CAD build for the part. Positions are in the model's coordinates, mm. A direction names the side the tool comes from. Coordinates: 2 decimals unless noted, no trailing zeros. Order: outer loops, then holes, each group sorted by start corner. A loop starts at its lowest first (then second) coordinate and runs counter-clockwise, first axis right, second up. Notation, with made-up numbers: M 23,57.25 L 40,57.25 A22 cw 40,76.25 Z; hole C 45.5,-1.75 d4. An arc over 180 degrees is marked long. One line per item, written item: value.
from build123d import *

# Parameters (mm, degrees)
SKETCH2_R                = 3.175
CUT_EXTRUDE1_DEPTH       = 6.715
CUT_EXTRUDE1_DEPTH_BACK  = 6.715
SKETCH3_R                = 5.715
SKETCH3_R_2              = 3.175
BOSS_EXTRUDE1_DEPTH      = 6.0325
BOSS_EXTRUDE1_DEPTH_BACK = 6.0325
SKETCH4_W                = 5.08
SKETCH4_H                = 5.08
BOSS_EXTRUDE2_DEPTH      = 25.4


with BuildPart() as part:
    # Sketch1 → Revolve1 (revolve)
    with BuildSketch(Plane.XY):
        with BuildLine():
            Line((0, 5.715), (0, -5.715))
            ThreePointArc((0, -5.715), (5.715, 0), (0, 5.715))
        make_face()
    revolve(axis=Axis((0, 5.715, 0), (0, -1, 0)))

    # Sketch2 → Cut-Extrude1 (cut, two sides)
    with BuildSketch(Plane(origin=(0, 0, 0), x_dir=(1, 0, 0), z_dir=(0, 1, 0))) as cut_extrude1_sk:
        Circle(SKETCH2_R)
    extrude(amount=CUT_EXTRUDE1_DEPTH, mode=Mode.SUBTRACT)
    extrude(cut_extrude1_sk.sketch, amount=-CUT_EXTRUDE1_DEPTH_BACK, mode=Mode.SUBTRACT)

    # Sketch3 → Boss-Extrude1 (add, two sides)
    with BuildSketch(Plane(origin=(0, 0, 0), x_dir=(1, 0, 0), z_dir=(0, 1, 0))) as boss_extrude1_sk:
        Circle(SKETCH3_R)
        Circle(SKETCH3_R_2, mode=Mode.SUBTRACT)
    extrude(amount=BOSS_EXTRUDE1_DEPTH)
    extrude(boss_extrude1_sk.sketch, amount=-BOSS_EXTRUDE1_DEPTH_BACK)

    # Sketch4 → Boss-Extrude2 (add)
    with BuildSketch(Plane(origin=(0, 0, 0), x_dir=(0, 0, -1), z_dir=(-0.993884104, 0.1104282, 0))):
        Rectangle(SKETCH4_W, SKETCH4_H)
    extrude(amount=-BOSS_EXTRUDE2_DEPTH)


solid = part.part
Q1. Slice it at D-D (y = 5.5). List the corners of the cut face in (x, z) (3 decimals).
Recorded:
outline: C 0,0 d11.43; hole C 0,0 d6.35
Q2. Which spindle directions (+Z, -Z, +X, -X, +Y, -Y) get a long thin tool onto all of the face, cutting with end or side? Do faces 1 (the face through (0, 0, 0)), 2 (the face through (1.423, -2.714, 0.036)), 3 (the face through (15, -2, 2.54)), 4 (the face through (15, -2, -2.54)), 5 (the face through (2.5, 6.032, 2.5)). Say none if no direction does.
Recorded:
face 1: +Y
face 2: -Y
face 3: +Z, +X, +Y, -Y
face 4: -Z, +X, +Y, -Y
face 5: +Z, -Z, +X, -X, +Y
Q3. Drill centre lines: line 1 along Z through (x, y) = (0, -1.5) (3 decimals); line 2 along Z through (x, y) = (0, 1.5) (3 decimals). Where is each one in solid material? Low to high.
Recorded:
line 1: z = -5.715 to -3.175, -2.54 to 2.54, 3.175 to 5.715
line 2: z = -5.715 to -3.175, 3.175 to 5.715
Q4. Slice it at C-C (x = -2). List the corners of the cut face in (y, z).
Recorded:
outline: M -6.03,-5.35 L 6.03,-5.35 L 6.03,-2.47 L -6.03,-2.47 Z; M -6.03,2.47 L 6.03,2.47 L 6.03,5.35 L -6.03,5.35 Z
Q5. Mould opens along Z. For faces 6 (the face through (-5.71, 0.08, -0.25)), 7 (the face through (1, 0, 2.54)), 8 (the face through (2.5, -6.032, 2.5)) say: released by +Z, released by -Z, zero draft, split by the parting line, or undercut.
Recorded:
face 6: split by the parting line
face 7: undercut
face 8: zero draft
Q6. Pin check, flat tips, straight feed: pin 1 Ø1.7 at (x, y) = (1, -0.5) entering from +Z; pin 2 Ø1 at (y, z) = (-2, -2.5) entering from -X; pin 3 Ø5 at (x, z) = (0, 0) entering from -Y; pin 4 Ø5 at (y, z) = (1, 2) entering from +X. Stop position of each tip, or through.
Recorded:
pin 1: stops at z = 5.71
pin 2: stops at x = -5.35
pin 3: stops at y = -2.83
pin 4: stops at x = 25.53
Q7. Slice it at B-B (z = 0). List the corners of the cut face in (x, y) (1 decimal).
Recorded:
outline: M -5.7,-6 L -3.2,-6 L -3.2,6 L -5.7,6 Z; M -0.3,-2.5 L 3.2,-2.9 L 3.2,-6 L 5.7,-6 L 5.7,-3.2 L 25,-5.3 L 25.5,-0.3 L 5.7,1.9 L 5.7,6 L 3.2,6 L 3.2,2.2 L 0.3,2.5 Z
Q8. Slice it at A-A (y = -4). List the corners of the cut face in (x, z) (3 decimals).
Recorded:
outline: C 0,0 d11.43; M 13,-2.54 L 25.112,-2.54 L 25.112,2.54 L 13,2.54 Z; hole C 0,0 d6.35
